Autodesk Inventor part; units mm, degrees
ref_plane "YZ Plane" through (0, 0, 0) normal (1, 0, 0) x (0, 1, 0)
ref_plane "XZ Plane" through (0, 0, 0) normal (0, 1, 0) x (-1, 0, 0)
ref_plane "XY Plane" through (0, 0, 0) normal (0, 0, 1) x (1, 0, 0)
sketch "Skizze1" plane through (0, 0, 0) normal (1, 0, 0) x (0, 1, 0)
  line L0 (11.4, 22.5) -> (11.4, 6.5)
  line L1 (11.4, 6.5) -> (16.4, 6.5)
  line L2 (16.4, 6.5) -> (16.4, 4)
  line L3 (16.4, 4) -> (11.4, 4)
  line L4 (11.4, 4) -> (11.4, 0)
  line L5 (11.4, 0) -> (0, 0)
  line L6 (0, 0) -> (0, 22.5)
  line L7 (0, 22.5) -> (11.4, 22.5)
  dimension "d0" = 2.5
  dimension "d1" = 5
  dimension "d2" = 4
  dimension "d3" = 16
  dimension "d4" = 11.4
extrude "Extrusion1" add sketch "Skizze1" along normal blind 12.3
mirror "Spiegeln1" about plane through (0, 0, 22.5) normal (0, -1, 0) of "Extrusion1"
sketch "Skizze2" plane through (12.3, 11.4, 0) normal (0, 0, -1) x (-1, 0, 0)
  circle A0 centre (6.15, -6.15) radius 6.15
  line L0 (12.3, 0) -> (0, 0)
  line L1 (6.15, 0) -> (6.15, -6.15) construction
  line L2 (6.15, -6.15) -> (12.3, -6.15) construction
  line L3 (12.3, 0) -> (12.3, -22.8) construction
  point P0 (12.3, -11.4)
extrude "Extrusion2" add sketch "Skizze2" along normal blind 4
sketch "Skizze3" plane through (6.15, 5.25, -4) normal (0, 0, -1) x (-1, 0, 0)
  arc A0 (-6.15, 0) -> (6.15, 0) centre (0, 0) ccw
  arc A1 (-2.9094, -5.4183) -> (2.9094, -5.4183) centre (0, -6.15) ccw
  point P0 (6.15, -5.25)
  dimension "d9" = 6
extrude "Extrusion3" add sketch "Skizze3" against normal up to surface (4 mm away)
sketch "Skizze4" plane through (0, 11.4, 4) normal (0, 0, -1) x (-1, 0, 0)
  line L0 (-12.3, -22.8) -> (-12.3, -27.8)
  line L1 (-12.3, 0) -> (-12.3, 5)
  line L2 (0, 5) -> (-12.3, 5)
  point P0 (0, -11.4)
  point P1 (-6.15, 2.5)
  point P2 (-6.15, -25.3)
  point P3 (-12.3, -25.3)
  point P4 (-12.3, 2.5)
  point P5 (-6.15, 5)
hole "Bohrung1" at (6.15, 13.9, 4) at (6.15, -13.9, 4) direction (0, 0, 1) diameter 3 end through all
sketch "Skizze5" plane through (12.3, 11.4, -4) normal (0, 0, -1) x (-1, 0, 0)
  circle A0 centre (6.15, -6.15) radius 2.25
  arc A1 (9.0594, -11.5683) -> (3.2406, -11.5683) centre (6.15, -6.15) ccw
  point P0 (12.3, -11.4)
  dimension "d19" = 4.5
extrude "Extrusion4" add sketch "Skizze5" along normal blind 4.5
sketch "Skizze6" plane through (0, 0, 0) normal (-1, 0, 0) x (0, 0, 1)
  line L0 (6.5, 11.4) -> (22.5, 11.4)
  line L1 (4, 16.4) -> (6.5, 16.4)
  line L2 (6.5, 16.4) -> (6.5, 11.4)
  line L3 (6.5, 11.4) -> (4, 11.4)
  line L4 (4, 11.4) -> (4, 16.4)
  point P0 (0, 0)
extrude "Extrusion5" cut sketch "Skizze6" against normal through all
properties part number "Motor"
Geometry check sheet. Reference: the model listing, model coordinates, mm. A direction names the side the tool comes from. Give positions to 0.01 mm unless a question says otherwise; leave off trailing zeros. Order: outer loops, then holes, each group sorted by start corner. A loop starts at its lowest first (then second) coordinate and runs counter-clockwise, first axis right, second up. Notation, with made-up numbers: (54, 32) - (61, 32) arc R27 ccw to (61, 55) - close; hole circle Ø9 at (22, 36.25). An arc over 180 degrees is marked (long way). Answer in a Markdown table with one row per item. Add a question column.
Q1. Cross-section at B-B, the plane x = 5. Enter the section's corners in (y, z).
Q2. Gauge pin test, flat ends, axial feed: pin 1 (5.5 mm diameter, centred on x = 8.5, y = -14.5, fed in from +Z); pin 2 (3 mm diameter, centred on x = 9.5, y = 8, fed in from -Z); pin 3 (5 mm diameter, centred on x = 5.5, y = -11, fed in from -Z); pin 4 (2.5 mm diameter, centred on x = 6.15, y = -13.9, fed in from +Z). Record the tip position at first contact, or that the pin passes through.
Q3. Cross-section at A-A, the plane y = -13.9. Enter the section's corners in (x, z).
Q4. Material ranges on probe 1 along Y at (x, z) = (6.15, 5.2); probe 2 along X at (y, z) = (-13.9, 5.4); probe 3 along Y at (x, z) = (6.5, 1), recorded low to high. Write a range as from..to.
Q5. Tool access check on faces 1 (the flat face through (6, 2, -4)), 2 (the flat face through (6, -12, 6.5)), 3 (the flat face through (6, -12, 4)), 4 (the flat face through (6, -7, 0)). Record the directions out of +Z, -Z, +X, -X, +Y, -Y that give a thin tool (end or side, any length) a straight path to the whole face; none if there is none.
Q6. Cross-section at C-C, the plane y = -0.9. Enter the section's corners in (x, z).
Q7. Cross-section at D-D, the plane z = 6. Enter the section's corners in (x, y), then the cut area to 3 significant figures.
Check values:
| question | item | result |
|---|---|---|
| 1 | outline | (-16.4, 4) - (-14.86, 4) - (-14.86, 6.5) - (-16.4, 6.5) - close; (-12.94, 4) - (-11.4, 4) - (-11.4, 0) - (-3.67, 0) - (-3.67, -4) - (3.32, -4) - (3.32, -8.5) - (7.18, -8.5) - (7.18, -4) - (11.29, -4) - (11.29, 0) - (11.4, 0) - (11.4, 22.5) - (-11.4, 22.5) - (-11.4, 6.5) - (-12.94, 6.5) - close |
| 2 | pin 1 | stops at z = 6.5 |
| 2 | pin 2 | stops at z = -4 |
| 2 | pin 3 | stops at z = 0 |
| 2 | pin 4 | passes through |
| 3 | outline | (0, 4) - (4.65, 4) - (4.65, 6.5) - (0, 6.5) - close; (7.65, 4) - (12.3, 4) - (12.3, 6.5) - (7.65, 6.5) - close |
| 4 | probe 1 | y = -16.4..-15.4, -12.4..11.4 |
| 4 | probe 2 | x = 0..4.65, 7.65..12.3 |
| 4 | probe 3 | y = -11.4..11.4 |
| 5 | face 1 | -Z |
| 5 | face 2 | +Z, +X, -X, -Y |
| 5 | face 3 | -Z, +X, -X, -Y |
| 5 | face 4 | -Z, -Y |
| 6 | outline | (0, 0) - (3.15, 0) - (3.15, -4) - (9.15, -4) - (9.15, 0) - (12.3, 0) - (12.3, 22.5) - (0, 22.5) - close |
| 7 | outline | (0, -16.4) - (12.3, -16.4) - (12.3, 11.4) - (0, 11.4) - close; hole circle Ø3 at (6.15, -13.9) |
| 7 | area | 335 mm^2 |
